The listing builds one solid part. Answer for the finished solid, in the listing's coordinates (mm). Give positions to 0.01 mm unless a question says otherwise; leave off trailing zeros. Order: outer loops, then holes, each group sorted by start corner. A loop starts at its lowest first (then second) coordinate and runs counter-clockwise, first axis right, second up. Notation, with made-up numbers: (10, -21.75) -> (18, -21.75) arc R21 ccw to (18, -14.75) -> close; hole circle Ø6 at (72.25, 82). An arc over 180 degrees is marked (long way). One line per question, with ' | ' between items. Start each with the question number.
```python
from build123d import *

# Parameters (mm, degrees)
CROQUIS1_W              = 180
CROQUIS1_H              = 16
SALIENTE_EXTRUIR1_DEPTH = 5
CROQUIS2_W              = 170
CROQUIS2_H              = 17.74
SALIENTE_EXTRUIR2_DEPTH = 5
CROQUIS3_R              = 1.5
CORTAR_EXTRUIR1_DEPTH   = 5
CROQUIS4_W              = 170
CROQUIS4_H              = 2
CORTAR_EXTRUIR2_DEPTH   = 94.741920185
CROQUIS5_W              = 170
CROQUIS5_H              = 1
CORTAR_EXTRUIR3_DEPTH   = 10


with BuildPart() as part:
    # Croquis1 → Saliente-Extruir1 (new body)
    with BuildSketch(Plane(origin=(0, 0, 0), x_dir=(1, 0, 0), z_dir=(0, 1, 0))):
        Rectangle(CROQUIS1_W, CROQUIS1_H)
    extrude(amount=SALIENTE_EXTRUIR1_DEPTH)

    # Croquis2 → Saliente-Extruir2 (add)
    with BuildSketch(Plane(origin=(0, 5, 0), x_dir=(1, 0, 0), z_dir=(0, 1, 0))):
        with Locations((0, 16.87)):
            Rectangle(CROQUIS2_W, CROQUIS2_H)
        with Locations((0, -16.87)):
            Rectangle(CROQUIS2_W, CROQUIS2_H)
    extrude(amount=-SALIENTE_EXTRUIR2_DEPTH)

    # Croquis3 → Cortar-Extruir1 (cut)
    with BuildSketch(Plane(origin=(0, 5, 0), x_dir=(1, 0, 0), z_dir=(0, 1, 0))):
        with Locations(Location((-87, 0, 0), (0, 0, 270))):
            Circle(CROQUIS3_R)
    cortar_extruir1 = extrude(amount=-CORTAR_EXTRUIR1_DEPTH, mode=Mode.SUBTRACT)

    # Simetría1: Cortar-Extruir1 across plane
    add(cortar_extruir1.mirror(Plane(origin=(0, 0, 0), x_dir=(0, 0, 1), z_dir=(1, 0, 0))), mode=Mode.SUBTRACT)

    # Croquis4 → Cortar-Extruir2 (cut, through all)
    with BuildSketch(Plane(origin=(0, 5, 0), x_dir=(1, 0, 0), z_dir=(0, 1, 0))):
        with Locations((0, -24.74)):
            Rectangle(CROQUIS4_W, CROQUIS4_H)
    extrude(amount=-CORTAR_EXTRUIR2_DEPTH, mode=Mode.SUBTRACT)

    # Croquis5 → Cortar-Extruir3 (cut)
    with BuildSketch(Plane(origin=(0, 5, 0), x_dir=(1, 0, 0), z_dir=(0, 1, 0))):
        with Locations((0, 25.24)):
            Rectangle(CROQUIS5_W, CROQUIS5_H)
    extrude(amount=-CORTAR_EXTRUIR3_DEPTH, mode=Mode.SUBTRACT)


solid = part.part
```
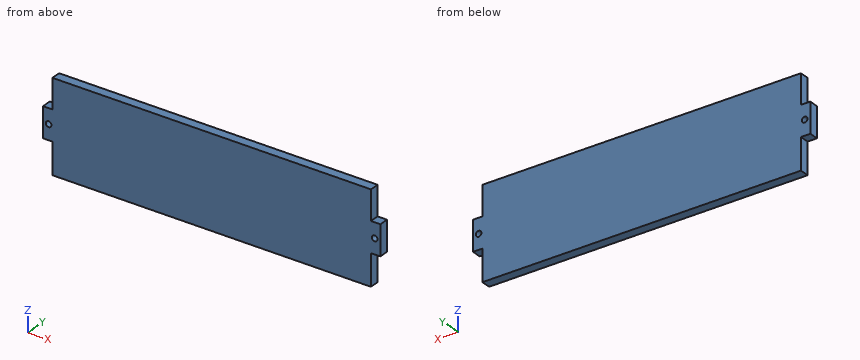
(1) Consider line 1 (X direction, y = 2.8, z = 0); line 2 (Z direction, x = -87, y = 1.95); line 3 (X direction, y = 3.5, z = 1). Determine where each line is inside the solid, lowest interval first.
(2) The part is cut by section C-C on y = 3.6. Determine the outline of the cut face in (x, z).
(3) The part is cut by section B-B on x = 87. Determine the outline of the cut face in (y, z).
(4) Given P1, Ø5, axis at x = -19.5, z = -16.5, coming from the -Y side; P2, Ø2.5, axis at y = 1.5, z = 15, coming from the +X side; P3, Ø1.5, axis at x = 86.5, y = 2.5, coming from the -Z side; P4, Ø2.5, axis at x = -88, y = 1.5, coming from the +Z side, each flat-ended and moving along its own axis, determine where each tip first touches the part or whether it passes through.
(5) The part is cut by section A-A on z = 0. Determine the outline of the cut face in (x, y).
(6) The part is cut by section D-D on z = 18.5. Determine the outline of the cut face in (x, y).
Result sheet:
1) line 1: x = -90 to -88.5, -85.5 to 85.5, 88.5 to 90 | line 2: z = -8 to -1.5, 1.5 to 8 | line 3: x = -90 to -88.12, -85.88 to 85.88, 88.12 to 90
2) outline: (-90, -8) -> (-85, -8) -> (-85, -24.74) -> (85, -24.74) -> (85, -8) -> (90, -8) -> (90, 8) -> (85, 8) -> (85, 23.74) -> (-85, 23.74) -> (-85, 8) -> (-90, 8) -> close; hole circle Ø3 at (-87, 0); hole circle Ø3 at (87, 0)
3) outline: (0, -8) -> (5, -8) -> (5, -1.5) -> (0, -1.5) -> close; (0, 1.5) -> (5, 1.5) -> (5, 8) -> (0, 8) -> close
4) P1: stops at y = 0 | P2: stops at x = 85 | P3: stops at z = -8 | P4: stops at z = 8
5) outline: (-90, 0) -> (-88.5, 0) -> (-88.5, 5) -> (-90, 5) -> close; (-85.5, 0) -> (85.5, 0) -> (85.5, 5) -> (-85.5, 5) -> close; (88.5, 0) -> (90, 0) -> (90, 5) -> (88.5, 5) -> close
6) outline: (-85, 0) -> (85, 0) -> (85, 5) -> (-85, 5) -> close
